```python
from build123d import *

# Parameters (mm, degrees)
SKETCH1_R           = 3
BOSS_EXTRUDE1_DEPTH = 1
SKETCH2_R           = 2
BOSS_EXTRUDE2_DEPTH = 5
SKETCH3_R           = 1
BOSS_EXTRUDE3_DEPTH = 6
SKETCH4_R           = 0.5
BOSS_EXTRUDE4_DEPTH = 0.5
FILLET2_R           = 0.5
SKETCH5_W           = 1
SKETCH5_H           = 1.914506357
BOSS_EXTRUDE5_DEPTH = 5
CIRPATTERN1_COUNT   = 3
SKETCH6_R           = 1.5
CUT_EXTRUDE1_DEPTH  = 5


with BuildPart() as part:
    # Sketch1 → Boss-Extrude1 (new body)
    with BuildSketch(Plane.XY):
        Circle(SKETCH1_R)
    extrude(amount=BOSS_EXTRUDE1_DEPTH)

    # Sketch2 → Boss-Extrude2 (add)
    with BuildSketch(Plane.XY.offset(1)):
        Circle(SKETCH2_R)
    extrude(amount=BOSS_EXTRUDE2_DEPTH)

    # Sketch3 → Boss-Extrude3 (add)
    with BuildSketch(Plane.XY.offset(6)):
        Circle(SKETCH3_R)
    extrude(amount=BOSS_EXTRUDE3_DEPTH)

    # Sketch4 → Boss-Extrude4 (add)
    with BuildSketch(Plane.XY.offset(12)):
        Circle(SKETCH4_R)
    extrude(amount=BOSS_EXTRUDE4_DEPTH)

    # Fillet2
    fillet2_edges = [part.edges().sort_by_distance(p)[0] for p in [
        (-0.5, 0, 12.5),
    ]]
    fillet(fillet2_edges, radius=FILLET2_R - 0.0001)  # a hair under: the kernel refuses the full size

    # Sketch5 → Boss-Extrude5 (add)
    with BuildSketch(Plane.XY.offset(1)):
        with Locations((0, 1.945455643)):
            Rectangle(SKETCH5_W, SKETCH5_H)
    boss_extrude5 = extrude(amount=BOSS_EXTRUDE5_DEPTH)

    # CirPattern1: Boss-Extrude5 ×3 about axis
    cirpattern1_axis = Axis((0, 0, 0), (0, 0, 1))
    for i in range(1, CIRPATTERN1_COUNT):
        add(boss_extrude5.rotate(cirpattern1_axis, i * 360 / CIRPATTERN1_COUNT))

    # Sketch6 → Cut-Extrude1 (cut)
    with BuildSketch(Plane(origin=(0, 0, 0), x_dir=(-1, 0, 0), z_dir=(0, 0, -1))):
        Circle(SKETCH6_R)
    extrude(amount=-CUT_EXTRUDE1_DEPTH, mode=Mode.SUBTRACT)


solid = part.part
```
Source: CAD feature listing. Evaluate the final solid. Frame: model axes, mm. A direction names the side the tool comes from. Round coordinates to 2 decimals unless told otherwise and drop trailing zeros. Loops run counter-clockwise (first coordinate to the right, second up) from the corner with the lowest first, then second, coordinate; pieces in that order, holes last. Notation, with made-up numbers: M 41.5,-3 L 69.5,-3 A24 ccw 69.5,25 Z; hole C 3,-27 d9. An arc over 180 degrees is marked long. Use a Markdown table: item, result. Add a question column.
1. Cut plane D-D, the plane x = -1.2. Output: boundary loops of the cut face in (y, z).
2. Cut plane C-C, the plane x = -2.6. Output: boundary loops of the cut face in (y, z).
3. Ray query, line 1 along X through (y, z) = (-1.6, 1.5); line 2 along Y through (x, z) = (0, 1.6); line 3 along X through (y, z) = (-1.55, 4.75). Return the intervals inside material, ascending. Write a range as [from, to].
4. Pull-direction query (Y, two-part tool) for faces 1 (the cylindrical face through (1.743, 0.981, 3.465)), 2 (the cylindrical face through (0, -2, 3)), 3 (the flat face through (-0.5, 2.4, 3.5)), 4 (the flat face through (0, 0, 5)); classes: +Y half, -Y half, draft (parallel to the pull), parting line (faces both ways), or undercut.
5. Set-up query: faces 5 (the flat face through (0, 2.903, 3)), 6 (the flat face through (-0.04, -1.15, 6)), 7 (the flat face through (2.517, -1.445, 3.465)), 8 (the flat face through (0.5, 2.4, 3.5)), 9 (the flat face through (-2.51, -1.46, 3.46)). Return all of +Z, -Z, +X, -X, +Y, -Y with unobstructed straight access to the full face (end or side cutting, diameter ignored); none if empty.
6. Cut plane B-B, the plane y = 0.75. Output: boundary loops of the cut face in (x, z), and give its area (3 significant figures).
7. Contact query for flat-ended pins moving along their axis: pin 1 (0.8 mm diameter, centred on y = 2, z = 2.5, fed in from -X); pin 2 (0.8 mm diameter, centred on x = 0, z = 4, fed in from +Y); pin 3 (3 mm diameter, centred on y = 1, z = 4, fed in from -X). Output: stop coordinate, or through.
8. Cut plane A-A, the plane z = 2.5. Output: boundary loops of the cut face in (x, y).
Solution:
| question | item | result |
|---|---|---|
| 1 | outline | M -2.75,0 L -0.9,0 L -0.9,5 L 0.9,5 L 0.9,0 L 2.75,0 L 2.75,1 L 1.6,1 L 1.6,6 L -1.6,6 L -1.6,1 L -2.75,1 Z |
| 2 | outline | M -1.5,0 L 1.5,0 L 1.5,1 L -0.92,1 L -0.92,6 L -1.3,6 L -1.3,1 L -1.5,1 Z |
| 3 | line 1 | x = [-2.43, -1.77], [-1.2, 1.2], [1.77, 2.43] |
| 3 | line 2 | y = [-2, -1.5], [1.5, 2.9] |
| 3 | line 3 | x = [-2.46, -1.68], [-1.26, 1.26], [1.68, 2.46] |
| 4 | face 1 | undercut |
| 4 | face 2 | -Y half |
| 4 | face 3 | draft |
| 4 | face 4 | undercut |
| 5 | face 5 | +Z, +X, -X, +Y |
| 5 | face 6 | +Z |
| 5 | face 7 | +Z, +X, -Y |
| 5 | face 8 | +Z, +X, +Y |
| 5 | face 9 | +Z, -X, -Y |
| 6 | outline | M -2.9,0 L -1.3,0 L -1.3,5 L 1.3,5 L 1.3,0 L 2.9,0 L 2.9,1 L 1.85,1 L 1.85,6 L 0.66,6 L 0.66,12 L -0.66,12 L -0.66,6 L -1.85,6 L -1.85,1 L -2.9,1 Z |
| 6 | area | 19.3 mm2 |
| 7 | pin 1 | stops at x = -1.2 |
| 7 | pin 2 | stops at y = 2.9 |
| 7 | pin 3 | stops at x = -2 |
| 8 | outline | M -2.76,-1.02 L -2.26,-1.88 L -1.43,-1.4 A2 ccw 1.43,-1.4 L 2.26,-1.88 L 2.76,-1.02 L 1.93,-0.54 A2 ccw 0.5,1.94 L 0.5,2.9 L -0.5,2.9 L -0.5,1.94 A2 ccw -1.93,-0.54 Z; hole C 0,0 d3 |
